Answer from the drawing. Dimensions are ordinates in mm from the lowest x, y and z of the part. A direction names the side the tool comes from. Coordinates: 2 decimals unless noted, no trailing zeros. Write each loop counter-clockwise with the first axis right and the second up, starting at its lowest first coordinate (ties: lowest second). Pieces come first, ordered by that corner, then holes.
1) Determine the mould class of the marked faces 1, 2 and 3 for opening direction X: +X half, -X half, draft (parallel to the pull), parting line (faces both ways), or undercut.
2) The part is cut by section A-A (x = 15). Determine the outline of the cut face in (y, z), then the cut area to 3 significant figures.
3) The part is cut by section D-D (z = 2.25). Determine the outline of the cut face in (x, y).
4) Find the intervals of material crossed by line 1 (X direction, y = 15, z = 26); line 2 (Y direction, x = 15, z = 3.2); line 3 (Z direction, x = 26, y = 3.5), in increasing order.
5) Which of the six approach directions +Z, -Z, +X, -X, +Y, -Y give full straight-line access (tool end or side, diameter ignored) to the marked faces 4 and 5?
6) The part is cut by section B-B (y = 15). Determine the outline of the cut face in (x, z), then the cut area to 3 significant figures.
7) The part is cut by section C-C (x = 26). Determine the outline of the cut face in (y, z).
8) This flat-tipped pin is pushed along its axis until it touches: pin 1 Ø8 at (y, z) = (15.5, 12.5) entering from -X. Where does it stop, or does it pass through?
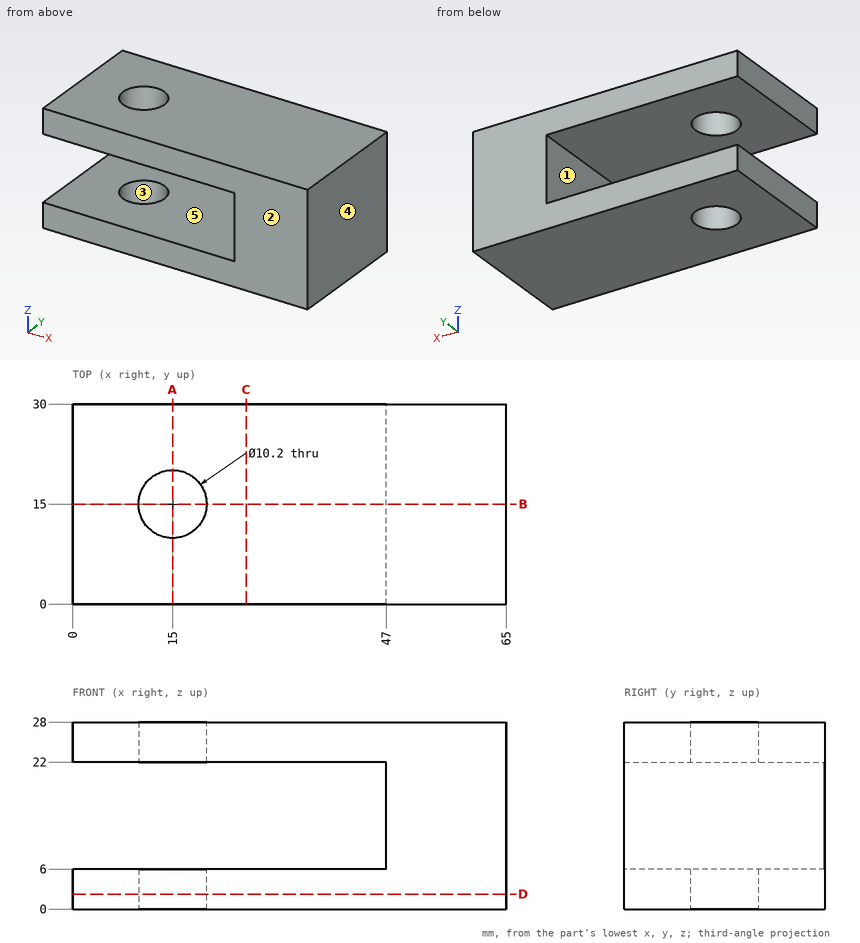
Reported:
1. face 1: -X half
1. face 2: draft
1. face 3: undercut
2. outline: (0, 0) - (9.9, 0) - (9.9, 6) - (0, 6) - close; (0, 22) - (9.9, 22) - (9.9, 28) - (0, 28) - close; (20.1, 0) - (30, 0) - (30, 6) - (20.1, 6) - close; (20.1, 22) - (30, 22) - (30, 28) - (20.1, 28) - close
2. area: 238 mm2
3. outline: (0, 0) - (65, 0) - (65, 30) - (0, 30) - close; hole circle Ø10.2 at (15, 15)
4. line 1: x = 0 to 9.9, 20.1 to 65
4. line 2: y = 0 to 9.9, 20.1 to 30
4. line 3: z = 0 to 6, 22 to 28
5. face 4: +Z, -Z, +X, +Y, -Y
5. face 5: -X, +Y, -Y
6. outline: (0, 0) - (9.9, 0) - (9.9, 6) - (0, 6) - close; (0, 22) - (9.9, 22) - (9.9, 28) - (0, 28) - close; (20.1, 0) - (65, 0) - (65, 28) - (20.1, 28) - (20.1, 22) - (47, 22) - (47, 6) - (20.1, 6) - close
6. area: 946 mm2
7. outline: (0, 0) - (30, 0) - (30, 6) - (0, 6) - close; (0, 22) - (30, 22) - (30, 28) - (0, 28) - close
8. pin 1: stops at x = 47
